Geometry: final body of the model. Coordinates: model frame, mm. A direction names the side the tool comes from. Round coordinates to 2 decimals unless told otherwise and drop trailing zeros. Loops run counter-clockwise (first coordinate to the right, second up) from the corner with the lowest first, then second, coordinate; pieces in that order, holes last. Notation, with made-up numbers: M 84,7.25 L 120,7.25 A17 ccw 120,39.25 Z; hole C 34,10 d7. An arc over 180 degrees is marked long. Return JSON: item names as keys, results as strings.
from build123d import *

# Parameters (mm, degrees)
SKETCH1_W           = 27.5
SKETCH1_H           = 30
SKETCH1_R           = 1.500000001
SKETCH1_R_2         = 1.5
BOSS_EXTRUDE1_DEPTH = 5
SKETCH1_3_W         = 7
SKETCH1_3_H         = 30
SKETCH1_3_R         = 1.500000001
SKETCH1_3_R_2       = 1.5
BOSS_EXTRUDE2_DEPTH = 15.6
SKETCH4_R           = 1.5
BOSS_EXTRUDE3_DEPTH = 4
BOSS_EXTRUDE4_START = -4
BOSS_EXTRUDE4_DEPTH = 3
SKETCH5_W           = 20.5
SKETCH5_H           = 30
CUT_EXTRUDE1_DEPTH  = 2


with BuildPart() as part:
    # Sketch1 → Boss-Extrude1 (new body)
    with BuildSketch(Plane.XY):
        with Locations((359.752910404, -328.295226576)):
            Rectangle(SKETCH1_W, SKETCH1_H)
        with Locations((370.002910404, -338.295226576)):
            Circle(SKETCH1_R, mode=Mode.SUBTRACT)
        with Locations((370.002910404, -318.295226576)):
            Circle(SKETCH1_R_2, mode=Mode.SUBTRACT)
        with Locations((350.002910404, -318.295226576)):
            Circle(SKETCH1_R_2, mode=Mode.SUBTRACT)
        with Locations((350.002910404, -338.295226576)):
            Circle(SKETCH1_R_2, mode=Mode.SUBTRACT)
    extrude(amount=BOSS_EXTRUDE1_DEPTH)

    # Sketch1<3> → Boss-Extrude2 (add)
    with BuildSketch(Plane.XY):
        with Locations((370.002910404, -328.295226576)):
            Rectangle(SKETCH1_3_W, SKETCH1_3_H)
        with Locations((370.002910404, -338.295226576)):
            Circle(SKETCH1_3_R, mode=Mode.SUBTRACT)
        with Locations((370.002910404, -318.295226576)):
            Circle(SKETCH1_3_R_2, mode=Mode.SUBTRACT)
    extrude(amount=BOSS_EXTRUDE2_DEPTH)

    # Sketch4 → Boss-Extrude3 (add)
    with BuildSketch(Plane(origin=(373.502910404, 0, 0), x_dir=(0, 0, -1), z_dir=(1, 0, 0))):
        Polygon((-15.6, -311.469542357), (-15.6, -313.295226576), (0, -313.295226576), (0, -311.469542357), (-2.5, -312.91291803), (-5.2, -311.354072303), (-5.2, -308.236380849), (-2.5, -306.677535123), (0, -308.120910796), (0, -306.295226576), (-15.6, -306.295226576), (-15.6, -308.120910796), (-13.1, -306.677535123), (-10.4, -308.236380849), (-10.4, -311.354072303), (-13.1, -312.91291803), align=None)
        Polygon((-2.5, -312.91291803), (0, -311.469542357), (0, -308.120910796), (-2.5, -306.677535123), (-5.2, -308.236380849), (-5.2, -311.354072303), align=None)
        with Locations((-2.5, -309.795226576)):
            Circle(SKETCH4_R, mode=Mode.SUBTRACT)
        Polygon((-15.6, -308.120910796), (-15.6, -311.469542357), (-13.1, -312.91291803), (-10.4, -311.354072303), (-10.4, -308.236380849), (-13.1, -306.677535123), align=None)
        with Locations((-13.1, -309.795226576)):
            Circle(SKETCH4_R, mode=Mode.SUBTRACT)
    boss_extrude3 = extrude(amount=-BOSS_EXTRUDE3_DEPTH)

    # Sketch4<3> → Boss-Extrude4 (add)
    with BuildSketch(Plane(origin=(373.502910404, 0, 0), x_dir=(0, 0, -1), z_dir=(1, 0, 0)).offset(BOSS_EXTRUDE4_START)):
        Polygon((-15.6, -311.469542357), (-15.6, -313.295226576), (0, -313.295226576), (0, -311.469542357), (-2.5, -312.91291803), (-5.2, -311.354072303), (-5.2, -308.236380849), (-2.5, -306.677535123), (0, -308.120910796), (0, -306.295226576), (-15.6, -306.295226576), (-15.6, -308.120910796), (-13.1, -306.677535123), (-10.4, -308.236380849), (-10.4, -311.354072303), (-13.1, -312.91291803), align=None)
    boss_extrude4 = extrude(amount=-BOSS_EXTRUDE4_DEPTH)

    # Mirror1: Boss-Extrude3, Boss-Extrude4 across plane
    add(boss_extrude3.mirror(Plane.ZX.offset(-328.295226576)))
    add(boss_extrude4.mirror(Plane.ZX.offset(-328.295226576)))

    # Sketch5 → Cut-Extrude1 (cut)
    with BuildSketch(Plane.XY.offset(5)):
        with Locations((356.252910404, -328.295226576)):
            Rectangle(SKETCH5_W, SKETCH5_H)
    extrude(amount=-CUT_EXTRUDE1_DEPTH, mode=Mode.SUBTRACT)


solid = part.part
Q1. Pull-direction query (Z, two-part tool) for faces 1 (the flat face through (368.02, -307.41, 14.37)), 2 (the flat face through (360, -328, 0)), 3 (the flat face through (370, -306.295, 8)); classes: pulls with the +Z half, pulls with the -Z half, needs draft (parallel to the pull), parting line crosses it, or undercut.
Determined:
{"face 1": "undercut", "face 2": "pulls with the -Z half", "face 3": "needs draft"}
Q2. Reachability of faces 4 (the flat face through (369.503, -308, 3)), 5 (the flat face through (356, -328, 3)), 6 (the cylindrical face through (371.53, -348.28, 13.3)), 7 (the flat face through (368, -347, 5.2)), 8 (the flat face through (370, -329, 15.6)) from +Z, -Z, +X, -X, +Y, -Y: full face, straight path, thin tool, end or side. Return the list, or none.
Determined:
{"face 4": "-X", "face 5": "+Z, -X, +Y, -Y", "face 6": "+X, -X", "face 7": "-Z, -X", "face 8": "+Z, +X, -X, +Y, -Y"}
Q3. Section query A-A (x = 370.5). Output: boundary loops of the cut face in (y, z).
Determined:
{"outline": "M -350.3,0 L -339.71,0 L -339.71,15.6 L -350.3,15.6 Z; M -336.88,0 L -319.71,0 L -319.71,15.6 L -336.88,15.6 Z; M -316.88,0 L -306.3,0 L -306.3,15.6 L -316.88,15.6 Z; hole C -346.8,2.5 d3; hole C -346.8,13.1 d3; hole C -309.8,2.5 d3; hole C -309.8,13.1 d3"}
Q4. Section query C-C (y = -340.5). Output: boundary loops of the cut face in (x, z), plus the area to 3 significant figures.
Determined:
{"outline": "M 346,0 L 373.5,0 L 373.5,15.6 L 366.5,15.6 L 366.5,3 L 346,3 Z", "area": "171 mm^2"}
Q5. Pin query (flat end, axial travel): pin 1 (2.5 mm diameter, centred on x = 370, y = -338.3, fed in from -Z); pin 2 (2.5 mm diameter, centred on x = 368, y = -346, fed in from +Z); pin 3 (4 mm diameter, centred on y = -309, z = 1.5, fed in from -X); pin 4 (1.5 mm diameter, centred on x = 355.5, z = 2, fed in from -Y). Return the tip coordinate at first contact, or that it passes through.
Determined:
{"pin 1": "passes through", "pin 2": "stops at z = 15.6", "pin 3": "stops at x = 366.5", "pin 4": "stops at y = -343.3"}
Q6. Section query D-D (x = 359.5). Output: boundary loops of the cut face in (y, z).
Determined:
{"outline": "M -343.3,0 L -313.3,0 L -313.3,3 L -343.3,3 Z"}
Q7. Material intervals for L1, parallel to Y at x = 370.5, z = 3.75; L2, parallel to Y at x = 368.75, z = 12.5; L3, parallel to Z at x = 347.5, y = -332, sorted ascending.
Determined:
{"L1": "y = -350.3 to -347.62, -345.97 to -339.71, -336.88 to -319.71, -316.88 to -310.62, -308.97 to -306.3", "L2": "y = -350.3 to -349.57, -344.02 to -339.12, -337.47 to -319.12, -317.47 to -312.57, -307.02 to -306.3", "L3": "z = 0 to 3"}
Q8. Section query B-B (z = 6.5). Output: boundary loops of the cut face in (x, y), plus the area to 3 significant figures.
Determined:
{"outline": "M 366.5,-350.3 L 373.5,-350.3 L 373.5,-306.3 L 366.5,-306.3 Z; hole C 370,-338.3 d3; hole C 370,-318.3 d3", "area": "294 mm^2"}
